```python
from build123d import *

# Parameters (mm, degrees)
SKETCH019_R  = 4
PAD008_DEPTH = 16.5
SKETCH020_R  = 5
PAD009_DEPTH = 5
FILLET001_R  = 0.25
FILLET002_R  = 0.5


with BuildPart() as part:
    # Sketch019 → Pad008 (new body)
    with BuildSketch(Plane(origin=(0, 0, 16.7), x_dir=(0, 1, 0), z_dir=(0, 0, 1))):
        Circle(SKETCH019_R)
    extrude(amount=PAD008_DEPTH)

    # Sketch020 (on Face3 of Pad008) → Pad009 (join)
    with BuildSketch(Plane(origin=(0, 0, 33.2), x_dir=(0, 1, 0), z_dir=(0, 0, 1))):
        Circle(SKETCH020_R)
    extrude(amount=PAD009_DEPTH)

    # Fillet001
    fillet001_edges = [part.edges().sort_by_distance(p)[0] for p in [
        (0, -5, 33.2),
    ]]
    fillet(fillet001_edges, radius=FILLET001_R)

    # Fillet002
    fillet002_edges = [part.edges().sort_by_distance(p)[0] for p in [
        (0, -5, 38.2),
    ]]
    fillet(fillet002_edges, radius=FILLET002_R)


solid = part.part
```
Geometry: final body of the model. Coordinates: model frame, mm. Round coordinates to 2 decimals unless told otherwise and drop trailing zeros. Order: outer loops, then holes, each group sorted by start corner. A loop starts at its lowest first (then second) coordinate and runs counter-clockwise, first axis right, second up. Notation, with made-up numbers: M -27,57.5 L -6,57.5 A21 ccw -6,96.5 Z; hole C 41,7 d11. An arc over 180 degrees is marked long. One line per item, written item: value.
(1) Pull-direction query (Z, two-part tool) for faces 1 (the flat face through (0, 0, 16.7)), 2 (the cylindrical face through (4.88, -1.08, 35.55)), 3 (the flat face through (0, 0, 38.2)); classes: pulls with the +Z half, pulls with the -Z half, needs draft (parallel to the pull), parting line crosses it, or undercut.
Result sheet:
face 1: pulls with the -Z half
face 2: needs draft
face 3: pulls with the +Z half
(2) Cut plane C-C (z = 34). Return the cut outline in (x, y), and give its area (3 significant figures).
Result sheet:
outline: C 0,0 d10
area: 78.5 mm2
(3) Line query: probe 1 along Z at (x, y) = (2.75, -3); probe 2 along X at (y, z) = (-3, 33.5); probe 3 along X at (y, z) = (-2.5, 19.5). Output: solid intervals per line, ascending. Write a range as [from, to].
Result sheet:
probe 1: [33.2, 38.2]
probe 2: [-4, 4]
probe 3: [-3.12, 3.12]
(4) Cut plane D-D (z = 31.25). Return the cut outline in (x, y), and give its area (3 significant figures).
Result sheet:
outline: C 0,0 d8
area: 50.3 mm2
(5) Cut plane A-A (y = 0). Return the cut outline in (x, z).
Result sheet:
outline: M -5,33.45 A0.25 ccw -4.75,33.2 L -4,33.2 L -4,16.7 L 4,16.7 L 4,33.2 L 4.75,33.2 A0.25 ccw 5,33.45 L 5,37.7 A0.5 ccw 4.5,38.2 L -4.5,38.2 A0.5 ccw -5,37.7 Z
(6) Pin query (flat end, axial travel): P1, Ø3, axis at x = -2, z = 27.5, coming from the -Y side; P2, Ø3, axis at x = 2, z = 33, coming from the +Y side. Return the tip coordinate at first contact, or that it passes through.
Result sheet:
P1: y = -3.97
P2: y = 4.97
